```python
from build123d import *

# Parameters (mm, degrees)
F0_R     = 16
F0_R_2   = 9.7
F1_DEPTH = 29
F2_R     = 9.75
F3_DEPTH = 12
F4_W     = 32
F4_H     = 6
F5_DEPTH = 25


with BuildPart() as f1:
    # F0 (on Top) → F1 (new body)
    with BuildSketch(Plane.XY):
        Circle(F0_R)
        Circle(F0_R_2, mode=Mode.SUBTRACT)
    extrude(amount=F1_DEPTH)

    # F2 (on Top) → F3 (join)
    with BuildSketch(Plane.XY):
        with BuildLine():
            Line((-16, 50), (-16, 0))
            ThreePointArc((-16, 0), (0, 16), (16, 0))
            Line((16, 0), (16, 50))
            Line((16, 50), (-16, 50))
        make_face()
        with BuildLine():
            ThreePointArc((16, 0), (0, 16), (-16, 0))
            ThreePointArc((-16, 0), (0, -16), (16, 0))
        make_face()
        Circle(F2_R, mode=Mode.SUBTRACT)
    extrude(amount=F3_DEPTH)

    # F4 (on face) → F5 (cut)
    with BuildSketch(Plane(origin=(0, 50, 0), x_dir=(-1, 0, 0), z_dir=(0, 1, 0))):
        with Locations((0, 6)):
            Rectangle(F4_W, F4_H)
    extrude(amount=-F5_DEPTH, mode=Mode.SUBTRACT)


solid = f1.part
```
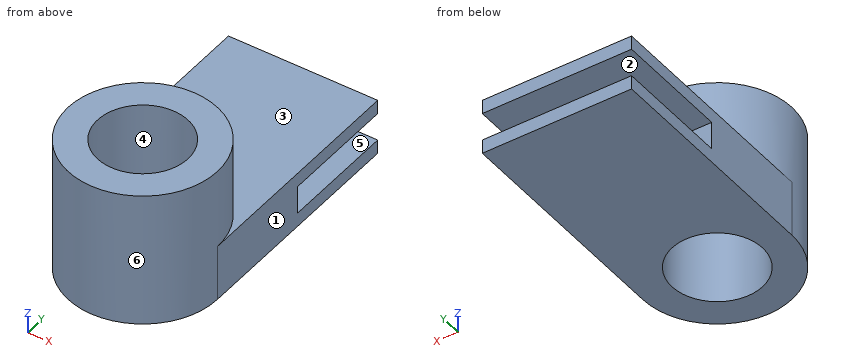
CAD build for the part. Positions are in the model's coordinates, mm. Face numbers are marked on the shaded views. A direction names the side the tool comes from. Give positions to 0.01 mm unless a question says otherwise; leave off trailing zeros. Order: outer loops, then holes, each group sorted by start corner. A loop starts at its lowest first (then second) coordinate and runs counter-clockwise, first axis right, second up. Notation, with made-up numbers: M 80,76.5 L 137,76.5 A14 cw 137,94.5 Z; hole C -30,66 d11. An arc over 180 degrees is marked long. Put each result on its own line as item: value. Start each with the question number.
(1) Saw through at B-B, the plane x = 0. Write the cut outline in (y, z).
(2) Flat gauge pins, fed straight in: pin 1 Ø1.8 at (x, z) = (-0.5, 6.5) entering from +Y; pin 2 Ø3 at (x, y) = (-4.5, 32.5) entering from +Z; pin 3 Ø2 at (x, z) = (2.5, 18) entering from -Y. Where does each tip first touch, or does it go through?
(3) Mould opens along Z. For the marked faces 1, 2 and 3 say: +Z half, -Z half, draft (parallel to the pull), parting line (faces both ways), or undercut.
(4) Drill centre lines: line 1 along Z through (x, y) = (-12.5, 41); line 2 along Y through (x, z) = (0, 22.75); line 3 along Y through (x, z) = (0, 10.5). Where is each one in solid material? Low to high.
(5) Saw through at A-A, the plane y = 31.5. Write the cut outline in (x, z).
(6) Saw through at C-C, the plane z = 20.5. Write the cut outline in (x, y), then the cut area to 3 significant figures.
(7) Saw through at D-D, the plane x = -11. Write the cut outline in (y, z), then the cut area to 3 significant figures.
(8) Which spindle directions (+Z, -Z, +X, -X, +Y, -Y) get a long thin tool onto all of the face, cutting with end or side? Do the marked faces 4, 5 and 6. Say none if no direction does.
Check result:
1. outline: M -16,0 L -9.7,0 L -9.7,29 L -16,29 Z; M 9.7,0 L 50,0 L 50,3 L 25,3 L 25,9 L 50,9 L 50,12 L 16,12 L 16,29 L 9.7,29 Z
2. pin 1: stops at y = 25
2. pin 2: stops at z = 12
2. pin 3: stops at y = -15.93
3. face 1: draft
3. face 2: undercut
3. face 3: +Z half
4. line 1: z = 0 to 3, 9 to 12
4. line 2: y = -16 to -9.7, 9.7 to 16
4. line 3: y = -16 to -9.7, 9.7 to 50
5. outline: M -16,0 L 16,0 L 16,3 L -16,3 Z; M -16,9 L 16,9 L 16,12 L -16,12 Z
6. outline: C 0,0 d32; hole C 0,0 d19.4
6. area: 509 mm2
7. outline: M -11.62,0 L 50,0 L 50,3 L 25,3 L 25,9 L 50,9 L 50,12 L 11.62,12 L 11.62,29 L -11.62,29 Z
7. area: 984 mm2
8. face 4: +Z, -Z
8. face 5: +X, -X, +Y
8. face 6: +Z
